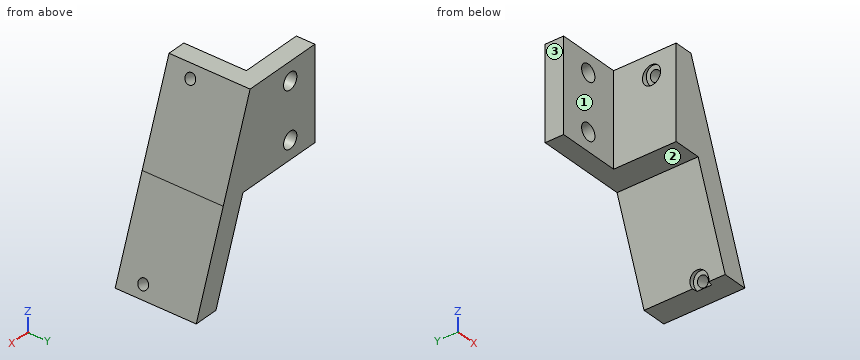
from build123d import *

# Parameters (mm, degrees)
BOSS_EXTRUDE1_DEPTH = 30
BOSS_EXTRUDE2_DEPTH = 26.3
BOSS_EXTRUDE3_DEPTH = 26.3
CUT_EXTRUDE1_REACH  = 58.563
SKETCH4_R           = 1.7
CUT_EXTRUDE2_START  = -6
SKETCH5_R           = 2.95
CUT_EXTRUDE2_DEPTH  = 21
SKETCH7_R           = 2.7
CUT_EXTRUDE3_DEPTH  = 21


with BuildPart() as part:
    # Sketch1 → Boss-Extrude1 (new body)
    with BuildSketch(Plane.XY):
        Polygon((0, 0), (0, 20.3), (-20.3, 20.3), (-20.3, 26.3), (6, 26.3), (6, 0), align=None)
    extrude(amount=BOSS_EXTRUDE1_DEPTH)

    # Sketch2 → Boss-Extrude2 (add)
    with BuildSketch(Plane.XZ):
        Polygon((6, 0), (16.919107028, 0), (6, 30), align=None)
    extrude(amount=-BOSS_EXTRUDE2_DEPTH)

    # Sketch3 → Boss-Extrude3 (add)
    with BuildSketch(Plane(origin=(0, 26.3, 0), x_dir=(1, 0, 0), z_dir=(0, 1, 0))):
        Polygon((16.919107028, 0), (27.889289173, 30.14032773), (19.889289173, 30.14032773), (8.919107028, 0), align=None)
    extrude(amount=-BOSS_EXTRUDE3_DEPTH)

    # Cut-Extrude1: up to this plane
    cut_extrude1_end = Plane(origin=(0, 0, 30), z_dir=(1, 0, 0))
    # Sketch4 → Cut-Extrude1 (cut, up to the surface)
    with BuildSketch(Plane(origin=(14.939947475, 0, 5.437696182), x_dir=(0.34202014332567265, 0, -0.9396926207859071), z_dir=(0.9396926207859071, 0, 0.34202014332567265)), mode=Mode.PRIVATE) as cut_extrude1_sk1:
        with Locations((-22.138657764, 8)):
            Circle(SKETCH4_R)
    cut_extrude1_tool1 = split(extrude(cut_extrude1_sk1.sketch, amount=-CUT_EXTRUDE1_REACH, mode=Mode.PRIVATE), bisect_by=cut_extrude1_end, keep=Keep.BOTH, mode=Mode.PRIVATE)
    add(cut_extrude1_tool1.solids().sort_by_distance((7.368081, 8, 26.24123))[0], mode=Mode.SUBTRACT)
    # Sketch4 → Cut-Extrude1 (cut, up to the surface)
    with BuildSketch(Plane(origin=(14.939947475, 0, 5.437696182), x_dir=(0.34202014332567265, 0, -0.9396926207859071), z_dir=(0.9396926207859071, 0, 0.34202014332567265)), mode=Mode.PRIVATE) as cut_extrude1_sk2:
        with Locations(Location((33.861342236, 8, 0), (0, 0, 41.975179766))):
            Circle(SKETCH4_R)
    cut_extrude1_tool2 = split(extrude(cut_extrude1_sk2.sketch, amount=-CUT_EXTRUDE1_REACH, mode=Mode.PRIVATE), bisect_by=cut_extrude1_end, keep=Keep.BOTH, mode=Mode.PRIVATE)
    add(cut_extrude1_tool2.solids().sort_by_distance((26.521209, 8, -26.381557))[0], mode=Mode.SUBTRACT)

    # Sketch5 → Cut-Extrude2 (cut)
    with BuildSketch(Plane(origin=(14.939947475, 0, 5.437696182), x_dir=(0.34202014332567265, 0, -0.9396926207859071), z_dir=(0.9396926207859071, 0, 0.34202014332567265)).offset(CUT_EXTRUDE2_START)):
        with Locations((-22.138657764, 8)):
            Circle(SKETCH5_R)
        with Locations((33.861342236, 8)):
            Circle(SKETCH5_R)
    extrude(amount=-CUT_EXTRUDE2_DEPTH, mode=Mode.SUBTRACT)

    # Sketch7 → Cut-Extrude3 (cut)
    with BuildSketch(Plane(origin=(0, 26.3, 0), x_dir=(1, 0, 0), z_dir=(0, 1, 0))):
        with Locations(Location((-10.3, -24, 0), (0, 0, 180))):
            Circle(SKETCH7_R)
        with Locations(Location((-10.3, -6, 0), (0, 0, 180))):
            Circle(SKETCH7_R)
    extrude(amount=-CUT_EXTRUDE3_DEPTH, mode=Mode.SUBTRACT)


solid = part.part
Verification items for the finished model (mm, model axes). Face numbers are marked on the shaded views. A direction names the side the tool comes from. Coordinates: 2 decimals unless noted, no trailing zeros. Order: outer loops, then holes, each group sorted by start corner. A loop starts at its lowest first (then second) coordinate and runs counter-clockwise, first axis right, second up.
Item 1: Section check D-D, the plane x = -17. Enter the section's corners in (y, z).
Filled in:
outline: (20.3, 0) - (26.3, 0) - (26.3, 30) - (20.3, 30) - close
Item 2: Section check C-C, the plane y = 4. Enter the section's corners in (x, z).
Filled in:
outline: (0, 0) - (8.92, 0) - (19.89, -30.14) - (27.89, -30.14) - (6, 30) - (0, 30) - close
Item 3: Section check A-A, the plane x = -10.3. Enter the section's corners in (y, z).
Filled in:
outline: (20.3, 0) - (26.3, 0) - (26.3, 3.3) - (20.3, 3.3) - close; (20.3, 8.7) - (26.3, 8.7) - (26.3, 21.3) - (20.3, 21.3) - close; (20.3, 26.7) - (26.3, 26.7) - (26.3, 30) - (20.3, 30) - close
Item 4: Depth check by flat-ended pin: pin 1 (13 mm diameter, centred on x = -4, y = 17.5, fed in from -Z); pin 2 (5 mm diameter, centred on x = -10.3, z = 24, fed in from +Y); pin 3 (2 mm diameter, centred on y = 18.5, z = 1.5, fed in from +X); pin 4 (12 mm diameter, centred on y = 8.5, z = 0.5, fed in from -X). Enter the tip coordinate at first touch or a pass-through.
Filled in:
pin 1: stops at z = 0
pin 2: passes through
pin 3: stops at x = 16.74
pin 4: stops at x = 0
Item 5: Access from +Z, -Z, +X, -X, +Y, -Y to the whole of each face (thin tool, end or side, straight path). Record for the marked faces 1, 2 and 3.
Filled in:
face 1: +Z, -Z, -X, -Y
face 2: -Z, -X, +Y, -Y
face 3: +Z, -Z, -X, +Y, -Y
Item 6: Section check B-B, the plane z = 6. Enter the section's corners in (x, y).
Filled in:
outline: (-20.3, 20.3) - (-13, 20.3) - (-13, 26.3) - (-20.3, 26.3) - close; (-7.6, 20.3) - (0, 20.3) - (0, 0) - (14.74, 0) - (14.74, 26.3) - (-7.6, 26.3) - close
Item 7: Material ranges on L1, parallel to Z at x = -10.3, y = 22.6; L2, parallel to Z at x = -12, y = 20.75; L3, parallel to Y at x = -11, z = 13.5, recorded low to high.
Filled in:
L1: z = 0 to 3.3, 8.7 to 21.3, 26.7 to 30
L2: z = 0 to 3.9, 8.1 to 21.9, 26.1 to 30
L3: y = 20.3 to 26.3
